Design review of the part built by this model. Coordinates are the model's own, in mm. A direction names the side the tool comes from. Round coordinates to 2 decimals unless told otherwise and drop trailing zeros. Order: outer loops, then holes, each group sorted by start corner. A loop starts at its lowest first (then second) coordinate and runs counter-clockwise, first axis right, second up. Notation, with made-up numbers: M 2,-28.5 L 57,-28.5 A20 ccw 57,-8.5 Z; hole C 65,3 d2. An arc over 180 degrees is marked long. Write each question's results on one line, items separated by ' | '. Start each with the question number.
Item 1: Take a section at A-A, the plane y = 12. Write out the cut boundary in (x, z), plus the area to 3 significant figures.
Item 2: The part is to be moulded in two halves that separate along X. For faces 5 (the cylindrical face through (29.48, 10.13, -53.04)), 6 (the flat face through (-115, 0, 1)), 7 (the flat face through (23.993, -2.958, -0.7)), say which applies: +X half, -X half, draft (parallel to the pull), parting line (faces both ways), or undercut.
Item 3: Wall thickness on line 1 (Z direction, x = -3.5, y = 14.5); line 2 (Y direction, x = 11, z = -35.5); line 3 (Z direction, x = -180, y = -3): over which ranges is each line inside the solid? List them lowest first. Write a range as [from, to].
Item 4: Machinability: for faces 1 (the flat face through (5, 0, -10)), 2 (the flat face through (-115, -3, -50)), 3 (the flat face through (-24, 15, 1)), 4 (the flat face through (-200, -3, 1)), which of the approach directions +Z, -Z, +X, -X, +Y, -Y give a long, thin tool a straight path to every point of the face, cutting with its end or side? Answer none if there is none.
Item 5: Clearance check with flat-ended pins moving along their axes: pin 1 (5 mm diameter, centred on y = 14.5, z = 19, fed in from +X); pin 2 (1.8 mm diameter, centred on x = -80.5, y = -2.5, fed in from -Z); pin 3 (12.5 mm diameter, centred on y = 11.5, z = 1.5, fed in from -X). State where each tip first meets the part, or that it passes through.
Item 6: Take a section at B-B, the plane z = -35. Write out the cut boundary in (x, y), plus the area to 3 significant figures.
Item 7: Take a section at D-D, the plane y = 32. Write out the cut boundary in (x, z), plus the area to 3 significant figures.
Item 8: Take a section at C-C, the plane x = -118. Write out the cut boundary in (y, z).
```python
from build123d import *

# Parameters (mm, degrees)
F1_DEPTH = 6
F2_W     = 74.469754
F2_H     = 42
F3_DEPTH = 6
F5_D     = 16
F7_DEPTH = 15


with BuildPart() as f1:
    # F0 (on Front) → F1 (new body)
    with BuildSketch(Plane.XZ):
        Polygon((0, 50), (-200, 50), (-200, -50), (0, -50), (47.323171, -50), align=None)
    extrude(amount=F1_DEPTH)

    # F2 (on face) → F3 (join)
    with BuildSketch(Plane(origin=(0, 0, -50), x_dir=(1, 0, 0), z_dir=(0, 0, -1))):
        with Locations((10.088294, -15)):
            Rectangle(F2_W, F2_H)
    extrude(amount=F3_DEPTH)

    # F5 (through all)
    with Locations(Plane.XY.offset(-50)):
        with Locations((23.134094, 15)):
            Hole(F5_D / 2)

    # F6 (on face) → F7 (join)
    with BuildSketch(Plane(origin=(0, 0, 0), x_dir=(-1, 0, 0), z_dir=(0, 1, 0))):
        Polygon((27.146583, 50), (21.146583, 50), (21.146583, -50), (25.706659, -50), (27.146583, -50), align=None)
    extrude(amount=F7_DEPTH)


solid = f1.part
```
Results list:
1) outline: M -27.15,-56 L 15.72,-56 L 15.72,-50 L -21.15,-50 L -21.15,50 L -27.15,50 Z; M 30.55,-56 L 47.32,-56 L 47.32,-50 L 30.55,-50 Z | area: 958 mm²
2) face 5: undercut | face 6: draft | face 7: +X half
3) line 1: [-56, -50] | line 2: [-6, 0] | line 3: [-50, 50]
4) face 1: +Z, +X, +Y | face 2: -Z, -X, +Y, -Y | face 3: +Z, +X, -X, +Y | face 4: +Z, -Z, -X, +Y, -Y
5) pin 1: x = -21.15 | pin 2: z = -50 | pin 3: x = -27.15
6) outline: M -200,-6 L 40.22,-6 L 40.22,0 L -21.15,0 L -21.15,15 L -27.15,15 L -27.15,0 L -200,0 Z | area: 1,530 mm²
7) outline: M -27.15,-56 L 47.32,-56 L 47.32,-50 L -27.15,-50 Z | area: 447 mm²
8) outline: M -6,-50 L 0,-50 L 0,50 L -6,50 Z
